```python
from build123d import *

# Parameters (mm, degrees)
EXTRUDE_1_DEPTH     = 3.5
CUT_EXTRUDE_START   = 3.5
SKETCH_2_R          = 1.75
SKETCH_2_R_2        = 1.5
CUT_EXTRUDE_1_DEPTH = 3.5
SKETCH_3_R          = 5
EXTRUDE_2_DEPTH     = 10
EXTRUDE_START       = 5
SKETCH_4_R          = 5
EXTRUDE_3_DEPTH     = 1.5
CUT_EXTRUDE_START_2 = -10
SKETCH_5_R          = 4
CUT_EXTRUDE_2_DEPTH = 15


with BuildPart() as part:
    # 草图1 → 凸台-拉伸1 (new body)
    with BuildSketch(Plane(origin=(0, 0, 0), x_dir=(1, 0, 0), z_dir=(0, 1, 0))):
        with BuildLine():
            Line((-9.219544457, 6), (9.219544457, 6))
            ThreePointArc((9.219544457, 6), (11, 0), (9.219544457, -6))
            Line((9.219544457, -6), (-9.219544457, -6))
            ThreePointArc((-9.219544457, -6), (-11, 0), (-9.219544457, 6))
        make_face()
    extrude(amount=EXTRUDE_1_DEPTH)

    # 草图2 → 切除-拉伸1 (cut)
    with BuildSketch(Plane(origin=(0, 0, 0), x_dir=(1, 0, 0), z_dir=(0, 1, 0)).offset(CUT_EXTRUDE_START)):
        with Locations(Location((8, 0, 0), (0, 0, 270))):
            Circle(SKETCH_2_R)
        with Locations(Location((-8, 0, 0), (0, 0, 270))):
            Circle(SKETCH_2_R_2)
    extrude(amount=-CUT_EXTRUDE_1_DEPTH, mode=Mode.SUBTRACT)

    # 草图3 → 凸台-拉伸2 (add)
    with BuildSketch(Plane(origin=(0, 0, 0), x_dir=(1, 0, 0), z_dir=(0, 1, 0))):
        with Locations(Location((0, 0, 0), (0, 0, 270))):
            Circle(SKETCH_3_R)
    extrude(amount=-EXTRUDE_2_DEPTH)

    # 草图4 → 凸台-拉伸3 (add)
    with BuildSketch(Plane(origin=(0, 0, 0), x_dir=(1, 0, 0), z_dir=(0, 1, 0)).offset(EXTRUDE_START)):
        with Locations(Location((0, 0, 0), (0, 0, 270))):
            Circle(SKETCH_4_R)
    extrude(amount=-EXTRUDE_3_DEPTH)

    # 草图5 → 切除-拉伸2 (cut)
    with BuildSketch(Plane(origin=(0, 0, 0), x_dir=(1, 0, 0), z_dir=(0, 1, 0)).offset(CUT_EXTRUDE_START_2)):
        with Locations(Location((0, 0, 0), (0, 0, 270))):
            Circle(SKETCH_5_R)
    extrude(amount=CUT_EXTRUDE_2_DEPTH, mode=Mode.SUBTRACT)


solid = part.part
```
Model file for the job. Use its own axes, mm. A direction names the side the tool comes from. Round coordinates to 2 decimals unless told otherwise and drop trailing zeros. Write each loop counter-clockwise with the first axis right and the second up, starting at its lowest first coordinate (ties: lowest second). Pieces come first, ordered by that corner, then holes. Notation, with made-up numbers: (19, -26) - (49, -26) arc R19 cw to (49, 11) - close; hole circle Ø7 at (23.5, 56.25). An arc over 180 degrees is marked (long way). One line per item, written item: value.
(1) Two-plate mould, pull along Z, no slides. Class faces 4 (the cylindrical face through (9.735, 1.774, -0.228)), 5 (the cylindrical face through (-4.88, -4.93, -1.08)), 6 (the flat face through (5.04, 3.5, 1.25)), 7 (the flat face through (0, 2, -6)): pulls with the +Z half, pulls with the -Z half, needs draft (parallel to the pull), parting line crosses it, or undercut.
Values follow:
face 4: undercut
face 5: parting line crosses it
face 6: needs draft
face 7: pulls with the -Z half
(2) Drop flat-ended pins along their axis: P1, Ø2, axis at x = -3.5, y = -5.5, coming from the -Z side; P2, Ø5, axis at y = -0.5, z = 3, coming from the +X side; P3, Ø6, axis at x = 8.5, z = 3.5, coming from the +Y side. Give the stop position or say it passes through.
Values follow:
P1: stops at z = -4.33
P2: stops at x = 10.99
P3: stops at y = 3.5
(3) 3-axis set-ups, long thin cutter, end or side, ignore diameter. For faces 1 (the flat face through (5.04, 0, 1.25)), 2 (the cylindrical face through (-3.905, -2.605, -0.867)), 3 (the cylindrical face through (-4.88, 4.26, -1.08)): which of +Z, -Z, +X, -X, +Y, -Y reach the whole face in a straight line?
Values follow:
face 1: -Y
face 2: +Y, -Y
face 3: +Y
(4) Cut at D-D, the plane z = -3.25. Give the cut face in (x, y), plus the area to 3 significant figures.
Values follow:
outline: (-10.51, 0) - (-3.8, 0) - (-3.8, -10) - (-2.33, -10) - (-2.33, 5) - (-3.8, 5) - (-3.8, 3.5) - (-10.51, 3.5) - close; (2.33, -10) - (3.8, -10) - (3.8, 0) - (10.51, 0) - (10.51, 3.5) - (3.8, 3.5) - (3.8, 5) - (2.33, 5) - close
area: 91.0 mm²
(5) Cut at A-A, the plane x = 0. Give the cut face in (y, z).
Values follow:
outline: (-10, -5) - (0, -5) - (0, -6) - (3.5, -6) - (3.5, -5) - (5, -5) - (5, -4) - (-10, -4) - close; (-10, 4) - (5, 4) - (5, 5) - (3.5, 5) - (3.5, 6) - (0, 6) - (0, 5) - (-10, 5) - close
(6) Cut at B-B, the plane y = 0.5. Give the cut face in (x, z), plus the area to 3 significant figures.
Values follow:
outline: (-9.22, -6) - (9.22, -6) arc R11 ccw to (9.22, 6) - (-9.22, 6) arc R11 ccw to start; hole circle Ø3 at (-8, 0); hole circle Ø8 at (0, 0); hole circle Ø3.5 at (8, 0)
area: 183 mm²
(7) Cut at C-C, the plane z = -1. Give the cut face in (x, y).
Values follow:
outline: (-10.95, 0) - (-9.12, 0) - (-9.12, 3.5) - (-10.95, 3.5) - close; (-6.88, 0) - (-4.9, 0) - (-4.9, -10) - (-3.87, -10) - (-3.87, 5) - (-4.9, 5) - (-4.9, 3.5) - (-6.88, 3.5) - close; (3.87, -10) - (4.9, -10) - (4.9, 0) - (6.56, 0) - (6.56, 3.5) - (4.9, 3.5) - (4.9, 5) - (3.87, 5) - close; (9.44, 0) - (10.95, 0) - (10.95, 3.5) - (9.44, 3.5) - close
(8) Wall check: probe 1 along X at (y, z) = (2.85, 0); probe 2 along X at (y, z) = (-7, 0); probe 3 along Y at (x, z) = (-6.25, -2.5). Give the ranges that are in metal, low to high.
Values follow:
probe 1: x = -11 to -9.5, -6.5 to -4, 4 to 6.25, 9.75 to 11
probe 2: x = -5 to -4, 4 to 5
probe 3: y = 0 to 3.5
